```python
from build123d import *

# Parameters (mm, degrees)
SKETCH1_R           = 8.89
BOSS_EXTRUDE1_DEPTH = 152.4
SKETCH2_W           = 1.113251556
SKETCH2_H           = 8.614313674
CUT_EXTRUDE1_DEPTH  = 153.917704011


with BuildPart() as part:
    # Sketch1 → Boss-Extrude1 (new body)
    with BuildSketch(Plane(origin=(0, 0, 0), x_dir=(1, 0, 0), z_dir=(0, 1, 0))):
        with Locations(Location((0, 0, 0), (0, 0, 90))):
            Circle(SKETCH1_R)
        Polygon((3.959468146, -6.858), (7.918936292, 0), (3.959468146, 6.858), (-3.959468146, 6.858), (-7.918936292, 0), (-3.959468146, -6.858), align=None, mode=Mode.SUBTRACT)
    extrude(amount=BOSS_EXTRUDE1_DEPTH)

    # Sketch2 → Cut-Extrude1 (cut, through all)
    with BuildSketch(Plane(origin=(0, 0, 0), x_dir=(-1, 0, 0), z_dir=(0, -1, 0))):
        with Locations((0, -8.353945441)):
            Rectangle(SKETCH2_W, SKETCH2_H)
    extrude(amount=-CUT_EXTRUDE1_DEPTH, mode=Mode.SUBTRACT)


solid = part.part
```
Geometry check sheet. Reference: the model listing, model coordinates, mm. A direction names the side the tool comes from. Coordinates: 2 decimals unless noted, no trailing zeros. Loops run counter-clockwise (first coordinate to the right, second up) from the corner with the lowest first, then second, coordinate; pieces in that order, holes last. Notation, with made-up numbers: (-5.75, 71.25) -> (28.25, 71.25) arc R31 ccw to (28.25, 103.25) -> close; hole circle Ø6 at (76, 49). An arc over 180 degrees is marked (long way). Put each result on its own line as item: value.
1) Thickness scan on line 1 (Z direction, x = 5.5, y = 94); line 2 (Z direction, x = 5, y = 53.5); line 3 (X direction, y = 104.5, z = 1.5). Record the ranges inside material, lowest first.
Result set:
line 1: z = -6.98 to -4.19, 4.19 to 6.98
line 2: z = -7.35 to -5.06, 5.06 to 7.35
line 3: x = -8.76 to -7.05, 7.05 to 8.76
2) Tool access check on faces 3 (the flat face through (-5.967, 75.133, 3.381)), 4 (the flat face through (0, 0, -7.2)). Record the directions out of +Z, -Z, +X, -X, +Y, -Y that give a thin tool (end or side, any length) a straight path to the whole face; none if there is none.
Result set:
face 3: +Y, -Y
face 4: +Z, -Z, +X, -X, -Y
3) Cross-section at B-B on z = 5. Record the boundary of the cut face in (x, y), plus the area to 3 significant figures.
Result set:
outline: (-7.35, 0) -> (-5.03, 0) -> (-5.03, 152.4) -> (-7.35, 152.4) -> close; (5.03, 0) -> (7.35, 0) -> (7.35, 152.4) -> (5.03, 152.4) -> close
area: 707 mm^2
4) Gauge pin test, flat ends, axial feed: pin 1 Ø4 at (y, z) = (88.5, -4.5) entering from +X; pin 2 Ø2 at (x, y) = (2.5, 51) entering from +Z; pin 3 Ø0.6 at (y, z) = (108.5, 8) entering from -X. Record the tip position at first contact, or that the pin passes through.
Result set:
pin 1: stops at x = 8.53
pin 2: stops at z = 8.76
pin 3: stops at x = -4.44
5) Release check for a two-part mould opening along Z. For faces 1 (the flat face through (5.9, 75.1, 3.5)), 2 (the flat face through (0, 152.4, -7.2)) record: released by +Z, released by -Z, zero draft, split by the parting line, or undercut.
Result set:
face 1: undercut
face 2: zero draft
6) Cross-section at A-A on y = 105. Record the boundary of the cut face in (x, z).
Result set:
outline: (-7.92, 0) -> (-3.96, 6.86) -> (-0.56, 6.86) -> (-0.56, 8.87) arc R8.89 ccw (long way) to (0.56, 8.87) -> (0.56, 6.86) -> (3.96, 6.86) -> (7.92, 0) -> (3.96, -6.86) -> (-3.96, -6.86) -> close
